Input: part model. Units: mm. Frame: model coordinates. Face numbers are marked on the shaded views. A direction names the side the tool comes from. Round coordinates to 2 decimals unless told otherwise and drop trailing zeros. Loops run counter-clockwise (first coordinate to the right, second up) from the corner with the lowest first, then second, coordinate; pieces in that order, holes last. Notation, with made-up numbers: M -30,32.25 L 20,32.25 A35 ccw 20,70.25 Z; hole C -16.75,53.25 d8. An arc over 180 degrees is marked long. Return JSON: item names as keys, results as strings. Group by question number.
1) Access query for the marked faces 1, 2 and 3. Directions: +Z, -Z, +X, -X, +Y, -Y. A direction counts if a zero-diameter tool reaches every point of the face in a straight line with its end or side. Return the directions, or none.
2) Section C-C (x = -25). Output: boundary loops of the cut face in (y, z).
3) Section A-A (x = 60). Output: boundary loops of the cut face in (y, z), plus the area to 3 significant figures.
4) Section B-B (x = 15). Count the separate pieces of the cut face and the enclosed holes in it, plus the area to 3 significant figures.
5) Mould query, pull axis X, two halves, no side actions, for the marked faces 4, 5, 6 and 7. Classes: +X half, -X half, draft (parallel to the pull), parting line (faces both ways), or undercut.
6) Material intervals for line 1 (X direction, y = 8, z = 49.5); line 2 (Y direction, x = 75.5, z = 29.4); line 3 (X direction, y = -8, z = 44), sorted ascending. Write a range as from..to.
7) Contact query for flat-ended pins moving along their axis: P1, Ø3, axis at x = 75.5, y = 15, coming from the -Z side; P2, Ø12, axis at x = 4, y = 3.5, coming from the +Z side; P3, Ø1.5, axis at x = 74, z = 26.5, coming from the +Y side; P4, Ø6, axis at y = 20, z = 23, coming from the -X side. Output: stop coordinate, or through.
8) Section D-D (z = 23.5). Output: boundary loops of the cut face in (x, y).
from build123d import *

# Parameters (mm, degrees)
SKETCH1_W                    = 90
SKETCH1_H                    = 40
SKETCH1_R                    = 7.6
BOSS_EXTRUDE1_DEPTH          = 80
SKETCH2_W                    = 30.5
SKETCH2_H                    = 40
CUT_EXTRUDE1_DEPTH           = 10
SKETCH3_W                    = 23.5
SKETCH3_H                    = 30.5
SKETCH3_H_2                  = 10
CUT_EXTRUDE2_DEPTH           = 46
CHAMFER1_SIZE                = 10
SKETCH4_W                    = 30.5
SKETCH4_H                    = 3
BOSS_EXTRUDE2_DEPTH          = 20
SKETCH5_R                    = 1.75
CUT_EXTRUDE3_DEPTH           = 20
SKETCH6_R                    = 6
CUT_EXTRUDE4_DEPTH           = 20
SKETCH8_W                    = 30.5
SKETCH8_H                    = 7
CUT_EXTRUDE5_DEPTH           = 1
CHAMFER3_SIZE                = 8
CHAMFER3_SIZE_2              = 11
CHAMFER4_SIZE                = 8
CHAMFER4_SIZE_2              = 45.370254557
SKETCH9_R                    = 1.75
CUT_EXTRUDE6_DEPTH           = 33
CUT_EXTRUDE7_DEPTH           = 13.25
EXTRUDE_THIN1_DEPTH          = 15
FILLET1_R                    = 10
CUT_EXTRUDE_THIN1_DEPTH      = 112.915146428
CUT_EXTRUDE_THIN1_DEPTH_BACK = 95
FILLET2_START                = 10
FILLET2_DEPTH                = 3
BOSS_EXTRUDE3_DEPTH          = 11
CUT_EXTRUDE_THIN2_START      = -6
CUT_EXTRUDE_THIN2_DEPTH      = 148.230308362
CUT_EXTRUDE_THIN3_START      = -11
SKETCH15_W                   = 32
SKETCH15_H                   = 4
CUT_EXTRUDE_THIN3_DEPTH      = 153.230308362
SKETCH16_R                   = 1.75
CUT_EXTRUDE8_DEPTH           = 15.99669
SKETCH17_W                   = 3
SKETCH17_H                   = 6
CUT_EXTRUDE9_DEPTH           = 11
SKETCH18_W                   = 23
SKETCH18_H                   = 30.465957047
CUT_EXTRUDE10_DEPTH          = 72
SKETCH19_R                   = 3
CUT_EXTRUDE11_DEPTH          = 22


with BuildPart() as part:
    # Sketch1 → Boss-Extrude1 (new body)
    with BuildSketch(Plane.XY):
        with Locations((25, 0)):
            Rectangle(SKETCH1_W, SKETCH1_H)
        Circle(SKETCH1_R, mode=Mode.SUBTRACT)
        with Locations((50, 0)):
            Circle(SKETCH1_R, mode=Mode.SUBTRACT)
    extrude(amount=BOSS_EXTRUDE1_DEPTH)

    # Sketch2 → Cut-Extrude1 (cut)
    with BuildSketch(Plane.ZY.offset(20)):
        with Locations((40, 0)):
            Rectangle(SKETCH2_W, SKETCH2_H)
    extrude(amount=-CUT_EXTRUDE1_DEPTH, mode=Mode.SUBTRACT)

    # Sketch3 → Cut-Extrude2 (cut)
    with BuildSketch(Plane(origin=(0, 20, 0), x_dir=(1, 0, 0), z_dir=(0, 1, 0))):
        with Locations((25, -40)):
            Rectangle(SKETCH3_W, SKETCH3_H)
        with Locations((25, -12.5)):
            Rectangle(SKETCH3_W, SKETCH3_H_2)
        with Locations((25, -67.5)):
            Rectangle(SKETCH3_W, SKETCH3_H_2)
    extrude(amount=-CUT_EXTRUDE2_DEPTH, mode=Mode.SUBTRACT)

    # Chamfer1
    chamfer1_edges = [part.edges().sort_by_distance(p)[0] for p in [
        (13.25, -20, 67.5),
        (13.25, -20, 12.5),
    ]]
    chamfer(chamfer1_edges, length=CHAMFER1_SIZE)

    # Sketch4 → Boss-Extrude2 (add)
    with BuildSketch(Plane.ZY.offset(10)):
        with Locations((40, 11.5)):
            Rectangle(SKETCH4_W, SKETCH4_H)
    extrude(amount=BOSS_EXTRUDE2_DEPTH)

    # Sketch5 → Cut-Extrude3 (cut)
    with BuildSketch(Plane(origin=(0, 13, 0), x_dir=(1, 0, 0), z_dir=(0, 1, 0))):
        with Locations(Location((-25, -31.5, 0), (0, 0, 180))):
            Circle(SKETCH5_R)
        with Locations(Location((-25, -48.5, 0), (0, 0, 180))):
            Circle(SKETCH5_R)
    extrude(amount=-CUT_EXTRUDE3_DEPTH, mode=Mode.SUBTRACT)

    # Sketch6 → Cut-Extrude4 (cut)
    with BuildSketch(Plane(origin=(0, 13, 0), x_dir=(1, 0, 0), z_dir=(0, 1, 0))):
        with Locations(Location((-16, -30.75, 0), (0, 0, 90))):
            Circle(SKETCH6_R)
        with Locations(Location((-16, -49.25, 0), (0, 0, 270))):
            Circle(SKETCH6_R)
    extrude(amount=-CUT_EXTRUDE4_DEPTH, mode=Mode.SUBTRACT)

    # Sketch8 → Cut-Extrude5 (cut)
    with BuildSketch(Plane.ZY.offset(10)):
        with Locations((40, 16.5)):
            Rectangle(SKETCH8_W, SKETCH8_H)
    extrude(amount=-CUT_EXTRUDE5_DEPTH, mode=Mode.SUBTRACT)

    # Chamfer3
    # the kernel refuses this chamfer: 11, 8 mm, written as the material it takes off along each edge
    with BuildSketch(Plane(origin=(-20, 48.396981056, 55.25), x_dir=(0, 0, 1), z_dir=(0, -1, 0))) as chamfer3_piece_1:
        Polygon((CHAMFER3_SIZE, 0), (0, -CHAMFER3_SIZE_2), (0, 0), align=None)
    extrude(amount=35.396981056, mode=Mode.SUBTRACT)
    with BuildSketch(Plane(origin=(-20, 13, 24.75), x_dir=(1, 0, 0), z_dir=(0, 1, 0))) as chamfer3_piece_2:
        Polygon((CHAMFER3_SIZE_2, 0), (0, CHAMFER3_SIZE), (0, 0), align=None)
    extrude(amount=35.396981056, mode=Mode.SUBTRACT)

    # Chamfer4
    # the kernel refuses this chamfer: 45.370254557, 8 mm, written as the material it adds along each edge
    with BuildSketch(Plane(origin=(-20, 13, 55.25), x_dir=(0, 0, 1), z_dir=(0, -1, 0))) as chamfer4_piece_1_section:
        Polygon((CHAMFER4_SIZE, 0), (0, CHAMFER4_SIZE_2), (0, 0), align=None)
    chamfer4_piece_1 = extrude(amount=3, mode=Mode.PRIVATE)
    chamfer4_piece_1 = split(chamfer4_piece_1, bisect_by=Plane(origin=(-30, 13, 55.25), z_dir=(1, 0, 0)), keep=Keep.TOP, mode=Mode.PRIVATE)
    add(chamfer4_piece_1)
    # the kernel refuses this chamfer: 45.370254557, 8 mm, written as the material it adds along each edge
    with BuildSketch(Plane(origin=(-20, 10, 24.75), x_dir=(0, 0, -1), z_dir=(0, 1, 0))) as chamfer4_2_piece_1_section:
        Polygon((CHAMFER4_SIZE, 0), (0, CHAMFER4_SIZE_2), (0, 0), align=None)
    chamfer4_2_piece_1 = extrude(amount=3, mode=Mode.PRIVATE)
    chamfer4_2_piece_1 = split(chamfer4_2_piece_1, bisect_by=Plane(origin=(-30, 10, 24.75), z_dir=(1, 0, 0)), keep=Keep.TOP, mode=Mode.PRIVATE)
    add(chamfer4_2_piece_1)

    # Sketch9 → Cut-Extrude6 (cut)
    with BuildSketch(Plane.ZY.offset(10)):
        with Locations(Location((40, -10, 0), (0, 0, 270))):
            Circle(SKETCH9_R)
    extrude(amount=-CUT_EXTRUDE6_DEPTH, mode=Mode.SUBTRACT)

    # Sketch10 → Cut-Extrude7 (cut)
    with BuildSketch(Plane(origin=(13.25, 0, 0), x_dir=(0, 0, -1), z_dir=(1, 0, 0))):
        Polygon((-40, -13.464101615), (-37, -11.732050808), (-37, -8.267949192), (-40, -6.535898385), (-43, -8.267949192), (-43, -11.732050808), align=None)
    extrude(amount=-CUT_EXTRUDE7_DEPTH, mode=Mode.SUBTRACT)

    # Sketch11 → Extrude-Thin1 (add)
    with BuildSketch(Plane(origin=(0, 20, 0), x_dir=(1, 0, 0), z_dir=(0, 1, 0))):
        with BuildLine():
            ThreePointArc((6.729729503, -35.51864706), (-1.958918458, -40), (6.729729503, -44.48135294))
            Line((6.729729503, -44.48135294), (6.149975329, -43.666561497))
            ThreePointArc((6.149975329, -43.666561497), (-0.958918458, -40), (6.149975329, -36.333438503))
            Line((6.149975329, -36.333438503), (6.729729503, -35.51864706))
        make_face()
    extrude(amount=EXTRUDE_THIN1_DEPTH)

    # Fillet1
    # the kernel refuses this fillet: 10 mm, written as the material it takes off along each edge
    with BuildSketch(Plane(origin=(-45, 20, 80), x_dir=(0, 0, -1), z_dir=(1, 0, 0)), Plane(origin=(95, -20, 80), x_dir=(0, 0, -1), z_dir=(-1, 0, 0)), Plane(origin=(95, -20, 0), x_dir=(0, 1, 0), z_dir=(-1, 0, 0)), Plane(origin=(-45, 20, 0), x_dir=(0, -1, 0), z_dir=(1, 0, 0))) as fillet1_piece_1:
        with BuildLine():
            CenterArc((FILLET1_R, -FILLET1_R), FILLET1_R, 90, 90)
            Line((0, -FILLET1_R), (0, 0))
            Line((0, 0), (FILLET1_R, 0))
        make_face()
    extrude(amount=140, mode=Mode.SUBTRACT)

    # Sketch12 → Cut-Extrude-Thin1 (cut, two sides: drawn at the far end of the back side and taken through both)
    with BuildSketch(Plane.XY.offset(80).offset(-CUT_EXTRUDE_THIN1_DEPTH_BACK)):
        Polygon((3.119310539, -0.5), (7.6, -0.5), (42.4, -0.5), (46.98201893, -0.5), (46.98201893, 0.5), (42.4, 0.5), (7.6, 0.5), (3.119310539, 0.5), align=None)
    extrude(amount=CUT_EXTRUDE_THIN1_DEPTH + CUT_EXTRUDE_THIN1_DEPTH_BACK, mode=Mode.SUBTRACT)

    # Fillet2: read off the stored shape, not the designer's step
    # Fillet2 outline → Fillet2 (add)
    with BuildSketch(Plane(origin=(0, 0, 0), x_dir=(1, 0, 0), z_dir=(0, 1, 0)).offset(FILLET2_START)):
        with BuildLine():
            ThreePointArc((-30, -61.486730193), (-22.679491924, -68.807238269), (-20, -78.807238269))
            Line((-20, -78.807238269), (-20, -63.25))
            Line((-20, -63.25), (-30, -61.486730193))
        make_face()
        with BuildLine():
            Line((-20, -16.75), (-20, -1.192761731))
            ThreePointArc((-20, -1.192761731), (-22.679491924, -11.192761731), (-30, -18.513269807))
            Line((-30, -18.513269807), (-20, -16.75))
        make_face()
    extrude(amount=FILLET2_DEPTH)

    # Sketch13 → Boss-Extrude3 (add)
    with BuildSketch(Plane(origin=(70, 0, 0), x_dir=(0, 0, -1), z_dir=(1, 0, 0))):
        with BuildLine():
            Line((-10, 20), (-32, 20))
            Line((-32, 20), (-32, -20))
            Line((-32, -20), (-10, -20))
            ThreePointArc((-10, -20), (-2.928932188, -17.071067812), (0, -10))
            Line((0, -10), (0, 10))
            ThreePointArc((0, 10), (-2.928932188, 17.071067812), (-10, 20))
        make_face()
        with BuildLine():
            Line((-48, -20), (-48, 20))
            Line((-48, 20), (-70, 20))
            ThreePointArc((-70, 20), (-77.071067812, 17.071067812), (-80, 10))
            Line((-80, 10), (-80, -10))
            ThreePointArc((-80, -10), (-77.071067812, -17.071067812), (-70, -20))
            Line((-70, -20), (-48, -20))
        make_face()
    extrude(amount=BOSS_EXTRUDE3_DEPTH)

    # Sketch14 → Cut-Extrude-Thin2 (cut)
    with BuildSketch(Plane(origin=(81, 0, 0), x_dir=(0, 0, -1), z_dir=(1, 0, 0)).offset(CUT_EXTRUDE_THIN2_START)):
        Polygon((0, 6), (-29.211170014, 6), (-29.211170014, 10), (-16.003311772, 12.306433224), (-4.745103337, 10.807010671), (-5.009141506, 8.824516321), (-15.962361409, 10.283319029), (-27.211170014, 8.318986477), (-27.211170014, 8), (0, 8), align=None)
    cut_extrude_thin2 = extrude(amount=CUT_EXTRUDE_THIN2_DEPTH, mode=Mode.SUBTRACT)

    # Sketch15 → Cut-Extrude-Thin3 (cut)
    with BuildSketch(Plane(origin=(81, 0, 0), x_dir=(0, 0, -1), z_dir=(1, 0, 0)).offset(CUT_EXTRUDE_THIN3_START)):
        with Locations((-16, -6)):
            Rectangle(SKETCH15_W, SKETCH15_H)
    cut_extrude_thin3 = extrude(amount=CUT_EXTRUDE_THIN3_DEPTH, mode=Mode.SUBTRACT)

    # Sketch16 → Cut-Extrude8 (cut)
    with BuildSketch(Plane.XY.offset(32)):
        with Locations((75.5, 15)):
            Circle(SKETCH16_R)
        with Locations((75.5, -15)):
            Circle(SKETCH16_R)
    cut_extrude8 = extrude(amount=-CUT_EXTRUDE8_DEPTH, mode=Mode.SUBTRACT)

    # Sketch17 → Cut-Extrude9 (cut)
    with BuildSketch(Plane(origin=(81, 0, 0), x_dir=(0, 0, -1), z_dir=(1, 0, 0))):
        with Locations((-27.043626223, 15)):
            Rectangle(SKETCH17_W, SKETCH17_H)
    cut_extrude9 = extrude(amount=-CUT_EXTRUDE9_DEPTH, mode=Mode.SUBTRACT)

    # Mirror1: Cut-Extrude9 across plane
    add(cut_extrude9.mirror(Plane.ZX), mode=Mode.SUBTRACT)

    # Sketch18 → Cut-Extrude10 (cut)
    with BuildSketch(Plane(origin=(0, 20, 0), x_dir=(1, 0, 0), z_dir=(0, 1, 0))):
        with Locations((51.74672632, -40.017021476)):
            Rectangle(SKETCH18_W, SKETCH18_H)
    extrude(amount=-CUT_EXTRUDE10_DEPTH, mode=Mode.SUBTRACT)

    # Mirror4: Cut-Extrude-Thin2, Cut-Extrude-Thin3 across plane
    add(cut_extrude_thin2.mirror(Plane(origin=(-0.025214783, 0, 39.991629957), x_dir=(0.9999998012339909, 0, 0.0006305013708499051), z_dir=(0.0006305013708499051, 0, -0.999999801233991))), mode=Mode.SUBTRACT)
    add(cut_extrude_thin3.mirror(Plane(origin=(-0.025214783, 0, 39.991629957), x_dir=(0.9999998012339909, 0, 0.0006305013708499051), z_dir=(0.0006305013708499051, 0, -0.999999801233991))), mode=Mode.SUBTRACT)

    # Mirror5: Cut-Extrude8 across plane
    add(cut_extrude8.mirror(Plane(origin=(-0.025214783, 0, 39.991629957), x_dir=(0.9999998012339909, 0, 0.0006305013708499051), z_dir=(0.0006305013708499051, 0, -0.999999801233991))), mode=Mode.SUBTRACT)

    # Sketch19 → Cut-Extrude11 (cut)
    with BuildSketch(Plane.XY.offset(80)):
        with Locations((75.5, 15)):
            Circle(SKETCH19_R)
        with Locations((75.5, -15)):
            Circle(SKETCH19_R)
    extrude(amount=-CUT_EXTRUDE11_DEPTH, mode=Mode.SUBTRACT)


solid = part.part
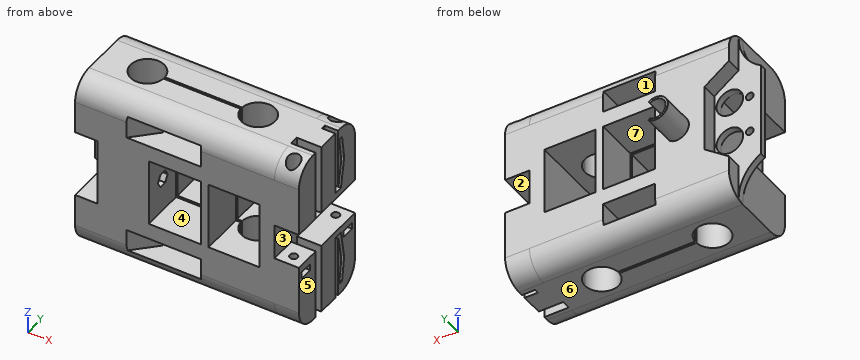
Returned:
{
 "1": {"face 1": "+Y, -Y", "face 2": "+X, +Y, -Y", "face 3": "+X"},
 "2": {"outline": "M 10,14.42 L 13,14.42 L 13,29.75 L 10,29.75 Z; M 10,33.25 L 13,33.25 L 13,46.75 L 10,46.75 Z; M 10,50.25 L 13,50.25 L 13,65.58 L 10,65.58 Z"},
 "3": {"outline": "M -20,10 A10 ccw -10,0 L 10,0 A10 ccw 20,10 L 20,24.78 L -20,24.78 Z; M -20,55.25 L 20,55.25 L 20,70 A10 ccw 10,80 L -10,80 A10 ccw -20,70 Z", "area": "1,900 mm^2"},
 "4": {"separate pieces": "8", "enclosed holes": "0", "area": "1,070 mm^2"},
 "5": {"face 4": "undercut", "face 5": "+X half", "face 6": "draft", "face 7": "undercut"},
 "6": {"line 1": "x = -10..13.25, 36.75..40.25, 63.25..81", "line 2": "y = -20..-16.75, -13.25..-8, -4..13.25, 16.75..20", "line 3": "x = -10..13.25, 36.75..40.25, 63.25..70"},
 "7": {"P1": "stops at z = 0.63", "P2": "stops at z = 80", "P3": "stops at y = 20", "P4": "stops at x = -15.53"},
 "8": {"outline": "M -30,10 L -20,10 L -20,-20 L 81,-20 L 81,-8 L 70,-8 L 70,-4 L 81,-4 L 81,6 L 75,6 L 75,8 L 81,8 L 81,8.97 L 75,8.97 L 75,11 L 81,11 L 81,20 L -10.72,20 L -10.72,13 L -30,13 Z; hole M 7.58,-0.5 L 42.42,-0.5 A7.6 ccw long 42.42,0.5 L 7.58,0.5 A7.6 ccw long Z; hole C 75.5,-15 d3.5; hole C 75.5,15 d3.5"}
}
